Input: part model. Units: mm. Frame: model coordinates. Give positions to 0.01 mm unless a question says otherwise; leave off trailing zeros. Order: outer loops, then holes, each group sorted by start corner. A loop starts at its lowest first (then second) coordinate and runs counter-clockwise, first axis right, second up.
```python
from build123d import *

# Parameters (mm, degrees)
MAINBODY_EXTRUDE_START                     = -15
MAINBODY_EXTRUDE_DEPTH                     = 30
VISESCREWSTHREADEDHOLES_CUT_DEPTH          = 23.101437038
VISESCREWSTHREADEDHOLES_CUT_DEPTH_BACK     = 23.101437038
VISESCREWSTHREADEDHOLES_SKETCH_R           = 2.1
CUT_EXTRUDE2_DEPTH                         = 24.435518325
CUT_EXTRUDE2_DEPTH_BACK                    = 19.935518325
CUT_EXTRUDE2_START                         = -4.5
THREADEDHOLEFORTERMINALSCREW_SKETCH_R      = 2.1
MOUNTINGHOLETOSIDEPLATESEEDFODDER_START    = -2.145727099
MOUNTINGHOLETOSIDEPLATESEEDFODDER_OUTLIN_W = 30
MOUNTINGHOLETOSIDEPLATESEEDFODDER_OUTLIN_H = 31.19125
MOUNTINGHOLETOSIDEPLATESEEDFODDER_OUTLIN_R = 2.1
MOUNTINGHOLETOSIDEPLATESEEDFODDER_DEPTH    = 2.645727099
MOUNTINGHOLETOSIDEPLATESEEDFODDER_START_2  = -15
MOUNTINGHOLETOSIDEPLATESEEDFODDER_2_DEPTH  = 30
MOUNTINGHOLETOSIDEPLATESEEDFODDER_START_3  = -4.5
MOUNTINGHOLETOSIDEPLATESEEDFODDER_3_OUTL_R = 2.1
MOUNTINGHOLETOSIDEPLATESEEDFODDER_3_DEPTH  = 9
MOUNTINGHOLETOSIDEPLATESEED_SKETCH_R       = 1.25
MOUNTINGHOLETOSIDEPLATESEED_CUT_DEPTH      = 23.101437038
MOUNTINGHOLESTOSIDEPLATE_PATTERN_START     = -15
MOUNTINGHOLESTOSIDEPLATE_PATTERN_OUTLINE_R = 1.25
MOUNTINGHOLESTOSIDEPLATE_PATTERN_DEPTH     = 30


with BuildPart() as part:
    # projectionX_sketch → mainBody_extrude (new body)
    with BuildSketch(Plane(origin=(0, 0, 0), x_dir=(0, 0, -1), z_dir=(1, 0, 0)).offset(MAINBODY_EXTRUDE_START)):
        with BuildLine():
            Line((-0.5, 15.595625), (2.145727099, 15.595625))
            ThreePointArc((2.145727099, 15.595625), (3.383636459, 15.399252271), (4.5, 14.829415207))
            Line((4.5, 14.829415207), (4.5, -15.595625))
            Line((4.5, -15.595625), (-4.5, -15.595625))
            Line((-4.5, -15.595625), (-4.5, 11.595625))
            ThreePointArc((-4.5, 11.595625), (-3.328427125, 14.424052125), (-0.5, 15.595625))
        make_face()
    extrude(amount=MAINBODY_EXTRUDE_DEPTH)

    # viseScrewsThreadedHoles_sketch → viseScrewsThreadedHoles_cut (cut, two sides: drawn at the far end of the back side and taken through both)
    with BuildSketch(Plane.XY.offset(-VISESCREWSTHREADEDHOLES_CUT_DEPTH_BACK)):
        with Locations((-5.25, 5.595625)):
            Circle(VISESCREWSTHREADEDHOLES_SKETCH_R)
        with Locations((5.25, 5.595625)):
            Circle(VISESCREWSTHREADEDHOLES_SKETCH_R)
    extrude(amount=VISESCREWSTHREADEDHOLES_CUT_DEPTH + VISESCREWSTHREADEDHOLES_CUT_DEPTH_BACK, mode=Mode.SUBTRACT)

    # threadedHoleForTerminalScrew_sketch → Cut-Extrude2 (cut, two sides: drawn at the far end of the back side and taken through both)
    with BuildSketch(Plane.XY.offset(4.5).offset(CUT_EXTRUDE2_START - CUT_EXTRUDE2_DEPTH_BACK)):
        with Locations((0, -6.404375)):
            Circle(THREADEDHOLEFORTERMINALSCREW_SKETCH_R)
    extrude(amount=CUT_EXTRUDE2_DEPTH + CUT_EXTRUDE2_DEPTH_BACK, mode=Mode.SUBTRACT)

    # mountingHolesToSidePlate_pattern: read off the stored shape, not the designer's step
    # mountingHolesToSidePlate_pattern outline → mountingHolesToSidePlate_pattern (cut)
    with BuildSketch(Plane.YZ.offset(MOUNTINGHOLESTOSIDEPLATE_PATTERN_START)):
        with Locations((-11.395625, 0)):
            Circle(MOUNTINGHOLESTOSIDEPLATE_PATTERN_OUTLINE_R)
        with Locations((11.395625, 0)):
            Circle(MOUNTINGHOLESTOSIDEPLATE_PATTERN_OUTLINE_R)
    extrude(amount=MOUNTINGHOLESTOSIDEPLATE_PATTERN_DEPTH, mode=Mode.SUBTRACT)


with BuildPart() as body_2:
    # mountingHoleToSidePlateSeedFodder: read off the stored shape, not the designer's step
    # mountingHoleToSidePlateSeedFodder outlin → mountingHoleToSidePlateSeedFodder (new body)
    with BuildSketch(Plane.XY.offset(MOUNTINGHOLETOSIDEPLATESEEDFODDER_START)):
        Rectangle(MOUNTINGHOLETOSIDEPLATESEEDFODDER_OUTLIN_W, MOUNTINGHOLETOSIDEPLATESEEDFODDER_OUTLIN_H)
        with Locations((0, -6.404375)):
            Circle(MOUNTINGHOLETOSIDEPLATESEEDFODDER_OUTLIN_R, mode=Mode.SUBTRACT)
        with Locations((-5.25, 5.595625)):
            Circle(MOUNTINGHOLETOSIDEPLATESEEDFODDER_OUTLIN_R, mode=Mode.SUBTRACT)
        with Locations((5.25, 5.595625)):
            Circle(MOUNTINGHOLETOSIDEPLATESEEDFODDER_OUTLIN_R, mode=Mode.SUBTRACT)
    extrude(amount=MOUNTINGHOLETOSIDEPLATESEEDFODDER_DEPTH)

    # mountingHoleToSidePlateSeedFodder 2 outl → mountingHoleToSidePlateSeedFodder 2 (add)
    with BuildSketch(Plane.YZ.offset(MOUNTINGHOLETOSIDEPLATESEEDFODDER_START_2)):
        with BuildLine():
            Line((15.595625, -2.145727099), (-15.595625, -2.145727099))
            Line((-15.595625, -2.145727099), (-15.595625, -4.5))
            Line((-15.595625, -4.5), (14.829415207, -4.5))
            ThreePointArc((14.829415207, -4.5), (15.399252271, -3.38363646), (15.595625, -2.145727099))
        make_face()
        with BuildLine():
            ThreePointArc((15.595625, 0.5), (14.424052125, 3.328427125), (11.595625, 4.5))
            Line((11.595625, 4.5), (-15.595625, 4.5))
            Line((-15.595625, 4.5), (-15.595625, 0.5))
            Line((-15.595625, 0.5), (15.595625, 0.5))
        make_face()
    extrude(amount=MOUNTINGHOLETOSIDEPLATESEEDFODDER_2_DEPTH)

    # mountingHoleToSidePlateSeedFodder 3 outl → mountingHoleToSidePlateSeedFodder 3 (cut)
    with BuildSketch(Plane.XY.offset(MOUNTINGHOLETOSIDEPLATESEEDFODDER_START_3)):
        with Locations((5.25, 5.595625)):
            Circle(MOUNTINGHOLETOSIDEPLATESEEDFODDER_3_OUTL_R)
        with Locations((-5.25, 5.595625)):
            Circle(MOUNTINGHOLETOSIDEPLATESEEDFODDER_3_OUTL_R)
        with Locations((0, -6.404375)):
            Circle(MOUNTINGHOLETOSIDEPLATESEEDFODDER_3_OUTL_R)
    extrude(amount=MOUNTINGHOLETOSIDEPLATESEEDFODDER_3_DEPTH, mode=Mode.SUBTRACT)

    # mountingHoleToSidePlateSeed_sketch → mountingHoleToSidePlateSeed_cut (cut, symmetric)
    with BuildSketch(Plane(origin=(0, 0, 0), x_dir=(0, 0, -1), z_dir=(1, 0, 0))):
        Circle(MOUNTINGHOLETOSIDEPLATESEED_SKETCH_R)
    extrude(amount=MOUNTINGHOLETOSIDEPLATESEED_CUT_DEPTH, both=True, mode=Mode.SUBTRACT)


solid = part.part
```
1) Cut plane D-D (x = 9.5). Return the cut outline in (y, z), then the cut area to 3 significant figures.
2) Cut plane C-C (y = 12). Return the cut outline in (x, z).
3) Cut plane A-A (x = -5.25). Return the cut outline in (y, z).
4) Line query: probe 1 along Y at (x, z) = (6.5, -0.25); probe 2 along X at (y, z) = (7, 1.5); probe 3 along X at (y, z) = (4, -0.25). Output: solid intervals per line, ascending.
5) First-contact query: P1, Ø2, axis at y = -11.4, z = 0, coming from the +X side; P2, Ø3, axis at y = 11.4, z = 0, coming from the -X side. Flat tips, straight axial feed; report the tip coordinate or a pass-through.
6) Pull-direction query (Y, two-part tool) for faces 1 (the face through (0, -15.596, 0)), 2 (the face through (-15, 0, 0)), 3 (the face through (-0.21, -12.644, 0.055)); classes: pulls with the +Y half, pulls with the -Y half, needs draft (parallel to the pull), parting line crosses it, or undercut.
7) Cut plane B-B (z = 0). Return the cut outline in (x, y).
Geometry says:
1. outline: (-15.6, -4.5) - (14.83, -4.5) arc R4 ccw to (15.6, -2.15) - (15.6, 0.5) arc R4 ccw to (11.6, 4.5) - (-15.6, 4.5) - close; hole circle Ø2.5 at (-11.4, 0); hole circle Ø2.5 at (11.4, 0)
1. area: 267 mm2
2. outline: (-15, -4.5) - (15, -4.5) - (15, -1.09) - (-15, -1.09) - close; (-15, 1.09) - (15, 1.09) - (15, 4.48) - (-15, 4.48) - close
3. outline: (-15.6, -4.5) - (3.5, -4.5) - (3.5, 4.5) - (-15.6, 4.5) - close; (7.7, -4.5) - (14.83, -4.5) arc R4 ccw to (15.6, -2.15) - (15.6, 0.5) arc R4 ccw to (11.6, 4.5) - (7.7, 4.5) - close; hole circle Ø2.5 at (-11.4, 0); hole circle Ø2.5 at (11.4, 0)
4. probe 1: y = -15.6 to -12.62, -10.17 to 3.91, 7.28 to 10.17, 12.62 to 15.6
4. probe 2: x = -15 to -6.81, -3.69 to 3.69, 6.81 to 15
4. probe 3: x = -15 to -6.62, -3.88 to 3.88, 6.62 to 15
5. P1: passes through
5. P2: stops at x = -15
6. face 1: pulls with the -Y half
6. face 2: needs draft
6. face 3: undercut
7. outline: (-15, -15.6) - (15, -15.6) - (15, -12.65) - (-15, -12.65) - close; (-15, -10.15) - (15, -10.15) - (15, 10.15) - (-15, 10.15) - close; (-15, 12.65) - (15, 12.65) - (15, 15.6) - (-15, 15.6) - close; hole circle Ø4.2 at (-5.25, 5.6); hole circle Ø4.2 at (0, -6.4); hole circle Ø4.2 at (5.25, 5.6)
